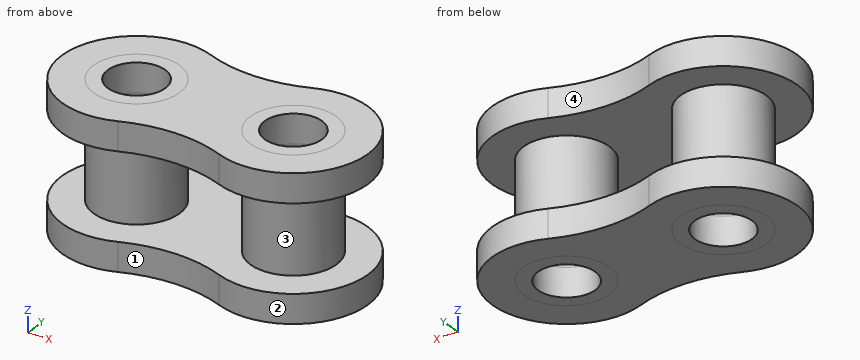
from build123d import *

# Parameters (mm, degrees)
SKETCH1_R           = 1
BOSS_EXTRUDE1_DEPTH = 1
BOSS_EXTRUDE2_START = -5
SKETCH2_R           = 1.5
SKETCH2_R_2         = 1
BOSS_EXTRUDE2_DEPTH = 5


with BuildPart() as part:
    # Sketch1 → Boss-Extrude1 (new body)
    with BuildSketch(Plane.XY):
        with BuildLine():
            ThreePointArc((-34.811060782, 2.411157676), (-38.383849898, 0), (-34.811060782, -2.411157676))
            ThreePointArc((-34.811060782, -2.411157676), (-33.033849898, -2.066157275), (-31.256639013, -2.411157676))
            ThreePointArc((-31.256639013, -2.411157676), (-27.683849898, 0), (-31.256639013, 2.411157676))
            ThreePointArc((-31.256639013, 2.411157676), (-33.033849898, 2.066157275), (-34.811060782, 2.411157676))
        make_face()
        with Locations((-35.783849898, 0)):
            Circle(SKETCH1_R, mode=Mode.SUBTRACT)
        with Locations((-30.283849898, 0)):
            Circle(SKETCH1_R, mode=Mode.SUBTRACT)
    extrude(amount=BOSS_EXTRUDE1_DEPTH)


with BuildPart() as body_2:
    # Mirror2: mirrored copy
    add(part.part.mirror(Plane(origin=(0, 0, -1.5), x_dir=(1, 0, 0), z_dir=(0, 0, -1))))


with BuildPart() as part_1:
    add(part.part)

    add(body_2.part)  # Boss-Extrude2 merges body 2
    # Sketch2 → Boss-Extrude2 (add)
    # profile 1 of 2: a face of its own
    with BuildSketch(Plane.XY.offset(1).offset(BOSS_EXTRUDE2_START)):
        with Locations((-30.283849898, 0)):
            Circle(SKETCH2_R)
        with Locations((-30.283849898, 0)):
            Circle(SKETCH2_R_2, mode=Mode.SUBTRACT)
    # profile 2 of 2: a face of its own
    with BuildSketch(Plane.XY.offset(1).offset(BOSS_EXTRUDE2_START)):
        with Locations((-35.783849898, 0)):
            Circle(SKETCH2_R)
        with Locations((-35.783849898, 0)):
            Circle(SKETCH2_R_2, mode=Mode.SUBTRACT)
    extrude(amount=BOSS_EXTRUDE2_DEPTH)


solid = part_1.part
Check sheet for the modelled part. Datum: model origin and axes. Units: mm. Face numbers are marked on the shaded views. A direction names the side the tool comes from. Give positions to 0.01 mm unless a question says otherwise; leave off trailing zeros. Loops run counter-clockwise (first coordinate to the right, second up) from the corner with the lowest first, then second, coordinate; pieces in that order, holes last. Notation, with made-up numbers: M 49.25,73 L 94.25,73 A25 cw 94.25,88 Z; hole C 6.5,77 d1. An arc over 180 degrees is marked long. Answer as a JSON object with one key per item and string values. Group by question number.
Q1. Material ranges on line 1 along Z through (x, y) = (-33.75, 0.75); line 2 along Y through (x, z) = (-30.25, -2.3); line 3 along Y through (x, z) = (-35.25, -0.35), recorded low to high. Write a range as [from, to].
Q2. Release check for a two-part mould opening along X. For the marked faces 1 and 2 record: released by +X, released by -X, zero draft, split by the parting line, or undercut.
Q3. Cross-section at C-C on y = -1.95. Record the cut outline in (x, z), then the cut area to 3 significant figures.
Q4. Cross-section at B-B on z = -0.65. Record the cut outline in (x, y), then the cut area to 3 significant figures.
Q5. Go/stop test with flat-tipped pins: P1, Ø1.2, axis at x = -30.28, y = 0, coming from the -Z side; P2, Ø2.5, axis at x = -35.78, y = 0, coming from the +Z side; P3, Ø3, axis at x = -32.5, z = -2, coming from the -Y side. Record where each tip stops, or that it passes through.
Q6. Cross-section at A-A on y = 0. Record the cut outline in (x, z), then the cut area to 3 significant figures.
Q7. Cross-section at D-D on x = -35. Record the cut outline in (y, z).
Q8. Access from +Z, -Z, +X, -X, +Y, -Y to the whole of each face (thin tool, end or side, straight path). Record for the marked faces 3 and 4.
Evaluation:
{
 "1": {"line 1": "z = [-4, -3], [0, 1]", "line 2": "y = [-1.5, -1], [1, 1.5]", "line 3": "y = [-1.4, -0.85], [0.85, 1.4]"},
 "2": {"face 1": "undercut", "face 2": "undercut"},
 "3": {"outline": "M -37.5,-4 L -28.56,-4 L -28.56,-3 L -37.5,-3 Z; M -37.5,0 L -28.56,0 L -28.56,1 L -37.5,1 Z", "area": "17.9 mm2"},
 "4": {"outline": "C -35.78,0 d3; C -30.28,0 d3; hole C -35.78,0 d2; hole C -30.28,0 d2", "area": "7.85 mm2"},
 "5": {"P1": "passes through", "P2": "stops at z = 1", "P3": "stops at y = -2.36"},
 "6": {"outline": "M -38.38,-4 L -36.78,-4 L -36.78,1 L -38.38,1 L -38.38,0 L -37.28,0 L -37.28,-3 L -38.38,-3 Z; M -34.78,-4 L -31.28,-4 L -31.28,1 L -34.78,1 Z; M -29.28,-4 L -27.68,-4 L -27.68,-3 L -28.78,-3 L -28.78,0 L -27.68,0 L -27.68,1 L -29.28,1 Z; hole M -34.28,-3 L -31.78,-3 L -31.78,0 L -34.28,0 Z", "area": "19.4 mm2"},
 "7": {"outline": "M -2.48,-4 L -0.62,-4 L -0.62,1 L -2.48,1 L -2.48,0 L -1.28,0 L -1.28,-3 L -2.48,-3 Z; M 0.62,-4 L 2.48,-4 L 2.48,-3 L 1.28,-3 L 1.28,0 L 2.48,0 L 2.48,1 L 0.62,1 Z"},
 "8": {"face 3": "none", "face 4": "+Z, -Z, +Y"}
}
